```python
from build123d import *

# Parameters (mm, degrees)
SKETCH_1_W      = 110
SKETCH_1_H      = 70
EXTRUDE_1_DEPTH = 20
SKETCH_2_R      = 5
EXTRUDE_2_DEPTH = 10


with BuildPart() as part:
    # 草图1 → 凸台-拉伸1 (new body)
    with BuildSketch(Plane.XY):
        Rectangle(SKETCH_1_W, SKETCH_1_H)
    extrude(amount=EXTRUDE_1_DEPTH)

    # 草图2 → 凸台-拉伸2 (add)
    with BuildSketch(Plane.ZY.offset(55)):
        with Locations(Location((9.669244668, 30, 0), (0, 0, 90))):
            Circle(SKETCH_2_R)
    extrude(amount=EXTRUDE_2_DEPTH)


solid = part.part
```
The listing builds one solid part. Answer for the finished solid, in the listing's coordinates (mm). A direction names the side the tool comes from. Coordinates: 2 decimals unless noted, no trailing zeros. Write each loop counter-clockwise with the first axis right and the second up, starting at its lowest first coordinate (ties: lowest second). Pieces come first, ordered by that corner, then holes. Notation, with made-up numbers: M 59,58 L 100,58 A23 cw 100,70 Z; hole C 81,89.5 d4. An arc over 180 degrees is marked long. Use a Markdown table: item, result. Add a question column.
1. Section B-B (z = 18.25) is taken. Give the vertices of the cut face in (x, y), plus the area to 3 significant figures.
2. Which of the six approach directions +Z, -Z, +X, -X, +Y, -Y give full straight-line access (tool end or side, diameter ignored) to faces 1 (the cylindrical face through (-59.93, 25.005, 9.449)), 2 (the flat face through (55, 0, 10))?
3. Section A-A (y = 30) is taken. Give the vertices of the cut face in (x, z).
4. Section C-C (y = -8.5) is taken. Give the vertices of the cut face in (x, z), plus the area to 3 significant figures.
5. Given P1, Ø1.5, axis at x = 16, y = -3.5, coming from the -Z side; P2, Ø6, axis at y = 12, z = 14, coming from the -X side, each flat-ended and moving along its own axis, determine where each tip first touches the part or whether it passes through.
6. A straight line is drawn through the part: line 1 along X through (y, z) = (20, 12). Find the intervals that lie inside material, in ascending order. Write a range as [from, to].
Data:
| question | item | result |
|---|---|---|
| 1 | outline | M -55,-35 L 55,-35 L 55,35 L -55,35 Z |
| 1 | area | 7,700 mm2 |
| 2 | face 1 | -X |
| 2 | face 2 | +Z, -Z, +X, +Y, -Y |
| 3 | outline | M -65,4.67 L -55,4.67 L -55,0 L 55,0 L 55,20 L -55,20 L -55,14.67 L -65,14.67 Z |
| 4 | outline | M -55,0 L 55,0 L 55,20 L -55,20 Z |
| 4 | area | 2,200 mm2 |
| 5 | P1 | stops at z = 0 |
| 5 | P2 | stops at x = -55 |
| 6 | line 1 | x = [-55, 55] |
